Build history of the part. All positions in model axes, mm. Give positions to 0.01 mm unless a question says otherwise; leave off trailing zeros. Order: outer loops, then holes, each group sorted by start corner. A loop starts at its lowest first (then second) coordinate and runs counter-clockwise, first axis right, second up. Notation, with made-up numbers: (55.25, 48.5) -> (73.25, 48.5) arc R22 cw to (73.25, 68.5) -> close; hole circle Ø11 at (-28, 78.25). An arc over 180 degrees is marked (long way). Use a Markdown table: item, result. Add a question column.
```python
from build123d import *

# Parameters (mm, degrees)
F0_W           = 103.1875
F0_H           = 19.05
F1_DEPTH       = 9.525
F2_R           = 3.175
F3_DEPTH       = 9.525
F5_D           = 6.35
F5_CSINK_D     = 9.525
F5_CSINK_ANGLE = 90


with BuildPart() as f1:
    # F0 (on Top) → F1 (new body)
    with BuildSketch(Plane.XY):
        with Locations((-5.027081, -9.736668)):
            Rectangle(F0_W, F0_H)
    extrude(amount=F1_DEPTH)

    # F2 (on face) → F3 (cut)
    with BuildSketch(Plane.XY.offset(9.525)):
        with BuildLine():
            ThreePointArc((-42.333331, -12.911668), (-45.508331, -9.736668), (-48.683331, -12.911668))
            ThreePointArc((-48.683331, -12.911668), (-45.508331, -16.086668), (-42.333331, -12.911668))
        make_face()
        with Locations((29.104169, -12.911668)):
            Circle(F2_R)
    extrude(amount=-F3_DEPTH, mode=Mode.SUBTRACT)

    # F5 (through all)
    with Locations(Plane(origin=(0, 0, 0), x_dir=(1, 0, 0), z_dir=(0, 0, -1))):
        with Locations((-45.508331, 12.911668), (29.104169, 12.911668)):
            CounterSinkHole(F5_D / 2, F5_CSINK_D / 2, counter_sink_angle=F5_CSINK_ANGLE)


solid = f1.part
```
(1) Mould opens along X. For faces 1 (the face through (-6, -10, 0)), 2 (the face through (-56.621, -10, 5)), 3 (the face through (-48.441, -11.696, 5.612)) say: released by +X, released by -X, zero draft, split by the parting line, or undercut.
(2) Band-saw the part on A-A on z = 3.5. Give the cut face in (x, y) (3 decimals).
(3) Wall check: probe 1 along X at (y, z) = (-12.75, 2.75); probe 2 along X at (y, z) = (-11.25, 8); probe 3 along Z at (x, y) = (-43, -10.5) (3 decimals). Give the ranges that are in metal, low to high.
(4) Band-saw the part on B-B on y = -14. State how many separate pieces and enclosed holes the cut face has, plus the area to 3 significant figures.
Response:
| question | item | result |
|---|---|---|
| 1 | face 1 | zero draft |
| 1 | face 2 | released by -X |
| 1 | face 3 | undercut |
| 2 | outline | (-56.621, -19.262) -> (46.567, -19.262) -> (46.567, -0.212) -> (-56.621, -0.212) -> close; hole circle Ø6.35 at (-45.508, -12.912); hole circle Ø6.35 at (29.104, -12.912) |
| 3 | probe 1 | x = -56.62 to -48.68, -42.34 to 25.93, 32.28 to 46.57 |
| 3 | probe 2 | x = -56.62 to -48.21, -42.8 to 26.4, 31.81 to 46.57 |
| 3 | probe 3 | z = 1.283 to 9.525 |
| 4 | separate pieces | 3 |
| 4 | enclosed holes | 0 |
| 4 | area | 864 mm² |
